Check sheet for the modelled part. Datum: model origin and axes. Units: mm. A direction names the side the tool comes from. Coordinates: 2 decimals unless noted, no trailing zeros. Write each loop counter-clockwise with the first axis right and the second up, starting at its lowest first coordinate (ties: lowest second). Pieces come first, ordered by that corner, then holes. Notation, with made-up numbers: M 62,74.25 L 118,74.25 A7 cw 118,84.25 Z; hole C 79,-31.5 d3. An arc over 180 degrees is marked long. Answer as CSV lines item,"result". Start each with the question number.
Q1. Depth check by flat-ended pin: pin 1 Ø0.6 at (x, z) = (-3, 0) entering from -Y; pin 2 Ø2 at (x, z) = (-2.5, -0.5) entering from +Y; pin 3 Ø1.6 at (x, y) = (0, 1.5) entering from -Z. Enter the tip coordinate at first touch or a pass-through.
Q2. Sectioned sample at A-A, the plane x = -2.5. Record the cut outline in (y, z), then the cut area to 3 significant figures.
Q3. Sectioned sample at C-C, the plane z = 0.75. Record the cut outline in (x, y).
Q4. Mould release check, pull along Z, two halves, no side actions. Record for faces 1 (the flat face through (2.056, 2, -2)), 2 (the flat face through (0, 2, 3.257)), 3 (the cylindrical face through (3.07, 3.18, 1.99)), 4 (the cylindrical face through (3.77, 2.46, 5.96)): pulls with the +Z half, pulls with the -Z half, needs draft (parallel to the pull), parting line crosses it, or undercut.
Q5. Sectioned sample at D-D, the plane x = 0.75. Record the cut outline in (y, z).
Q6. Sectioned sample at B-B, the plane z = -4. Record the cut outline in (x, y), then the cut area to 3 significant figures.
Q7. Access from +Z, -Z, +X, -X, +Y, -Y to the whole of each face (thin tool, end or side, straight path). Record for faces 5 (the cylindrical face through (3.07, 2.8, -4.696)), 6 (the flat face through (-3, 4.5, -1.743)), 7 (the cylindrical face through (-1.643, 2.465, 2.972)), 8 (the flat face through (-3, 0.5, 1.257)), 9 (the cylindrical face through (-3.643, 2.465, 5.972)).
Q8. Thickness scan on line 1 along X through (y, z) = (3.5, -4.5); line 2 along X through (y, z) = (0.6, -1.5); line 3 along X through (y, z) = (2.45, -4.5). Record the ranges inside material, lowest first. Write a range as from..to.
Autodesk Inventor part; units mm, degrees
ref_plane "YZ Plane" through (0, 0, 0) normal (1, 0, 0) x (0, 1, 0)
ref_plane "XZ Plane" through (0, 0, 0) normal (0, 1, 0) x (-1, 0, 0)
ref_plane "XY Plane" through (0, 0, 0) normal (0, 0, 1) x (1, 0, 0)
sketch "Sketch1" plane through (0, 0, 0) normal (0, 1, 0) x (-1, 0, 0)
  line L0 (-4.0561, -5.7426) -> (-4.0561, 5.2574)
  line L1 (-3.0561, 6.2574) -> (2.9439, 6.2574)
  line L2 (3.9439, 5.2574) -> (3.9439, -5.7426)
  line L3 (3.9439, -5.7426) -> (1.9439, -5.7426)
  line L4 (1.9439, -5.7426) -> (1.9439, 2.2574)
  line L5 (0.9439, 3.2574) -> (-1.0561, 3.2574)
  line L6 (-2.0561, 2.2574) -> (-2.0561, -5.7426)
  line L7 (-2.0561, -5.7426) -> (-4.0561, -5.7426)
  arc A0 (-1.0561, 3.2574) -> (-2.0561, 2.2574) centre (-1.0561, 2.2574) ccw
  arc A1 (1.9439, 2.2574) -> (0.9439, 3.2574) centre (0.9439, 2.2574) ccw
  arc A2 (-3.0561, 6.2574) -> (-4.0561, 5.2574) centre (-3.0561, 5.2574) ccw
  arc A3 (3.9439, 5.2574) -> (2.9439, 6.2574) centre (2.9439, 5.2574) ccw
  point P0 (0, 0)
  point P1 (-4.0561, 6.2574)
  point P2 (3.9439, 6.2574)
  point P3 (1.9439, 3.2574)
  point P4 (-2.0561, 3.2574)
  dimension "d0" = 12
  dimension "d1" = 2
  dimension "d2" = 2
  dimension "d3" = 8
  dimension "d4" = 3
  dimension "d20" = 1
extrude "Extrusion1" add sketch "Sketch1" along normal blind 5
sketch "Sketch2" plane through (4.0561, 0, 6.2574) normal (1, 0, 0) x (0, 0, -1)
  circle A0 centre (10, 2.5) radius 1
  circle A1 centre (5, 2.5) radius 1
  line L0 (12, 0) -> (12, 5)
  line L1 (1, 5) -> (12, 5)
  point P0 (6.2574, 0)
  point P1 (0, 5)
  dimension "d7" = 2
  dimension "d8" = 2
  dimension "d9" = 2
  dimension "d10" = 2.5
  dimension "d11" = 2.5
  dimension "d12" = 5
extrude "Extrusion2" cut sketch "Sketch2" against normal up to surface (2 mm away)
sketch "Sketch3" plane through (-3.9439, 0, -5.7426) normal (-1, 0, 0) x (0, 0, 1)
  line L0 (7, 0.0877) -> (7, 1)
  line L1 (7, 1) -> (4, 1)
  line L2 (4, 1) -> (4, 0)
  line L3 (0, 0) -> (11, 0)
  line L4 (11, 5) -> (0, 5)
  line L5 (7, 5) -> (7, 4)
  line L6 (7, 4) -> (4, 4)
  line L7 (4, 4) -> (4, 5)
  line L8 (7, 0.0877) -> (7, 0)
  line L9 (0, 0) -> (0, 5)
  point P0 (5.7426, 0)
  point P1 (12, 0)
  point P2 (12, 5)
  dimension "d15" = 1
  dimension "d16" = 1
  dimension "d17" = 3
  dimension "d21" = 4
extrude "Extrusion3" cut sketch "Sketch3" against normal up to next
properties part number "crochet"
Output:
1,pin 1,"stops at y = 1"
1,pin 2,"stops at y = 4"
1,pin 3,"stops at z = 3.26"
2,outline,"M 0,-5.74 L 5,-5.74 L 5,-1.74 L 4,-1.74 L 4,1.26 L 5,1.26 L 5,6.26 L 0,6.26 L 0,1.26 L 1,1.26 L 1,-1.74 L 0,-1.74 Z"
2,area,"54.0 mm^2"
3,outline,"M -3.94,1 L -1.94,1 L -1.94,4 L -3.94,4 Z; M 2.06,0 L 4.06,0 L 4.06,1.64 L 2.06,1.64 Z; M 2.06,3.36 L 4.06,3.36 L 4.06,5 L 2.06,5 Z"
4,face 1,"needs draft"
4,face 2,"pulls with the -Z half"
4,face 3,"undercut"
4,face 4,"pulls with the +Z half"
5,outline,"M 0,3.26 L 5,3.26 L 5,6.26 L 0,6.26 Z"
6,outline,"M -3.94,0 L -1.94,0 L -1.94,5 L -3.94,5 Z; M 2.06,0 L 4.06,0 L 4.06,1.53 L 2.06,1.53 Z; M 2.06,3.47 L 4.06,3.47 L 4.06,5 L 2.06,5 Z"
6,area,"16.1 mm^2"
7,face 5,"+X"
7,face 6,"-X, +Y"
7,face 7,"-Z, +Y, -Y"
7,face 8,"-X, -Y"
7,face 9,"+Z, -X, +Y, -Y"
8,line 1,"x = -3.94..-1.94, 2.06..4.06"
8,line 2,"x = 2.06..4.06"
8,line 3,"x = -3.94..-1.94"
